Can you work these out from the drawing? Everything is in mm from the part's minimum corner. A direction names the side the tool comes from. Coordinates: 2 decimals unless noted, no trailing zeros. Loops run counter-clockwise (first coordinate to the right, second up) from the corner with the lowest first, then second, coordinate; pieces in that order, holes last. Notation, with made-up numbers: M -31.75,-37 L -9.75,-37 A11 ccw -9.75,-30 Z; hole C -7,36.5 d1. An arc over 180 degrees is marked long. Write each question's results on one line, items separated by ' | '.
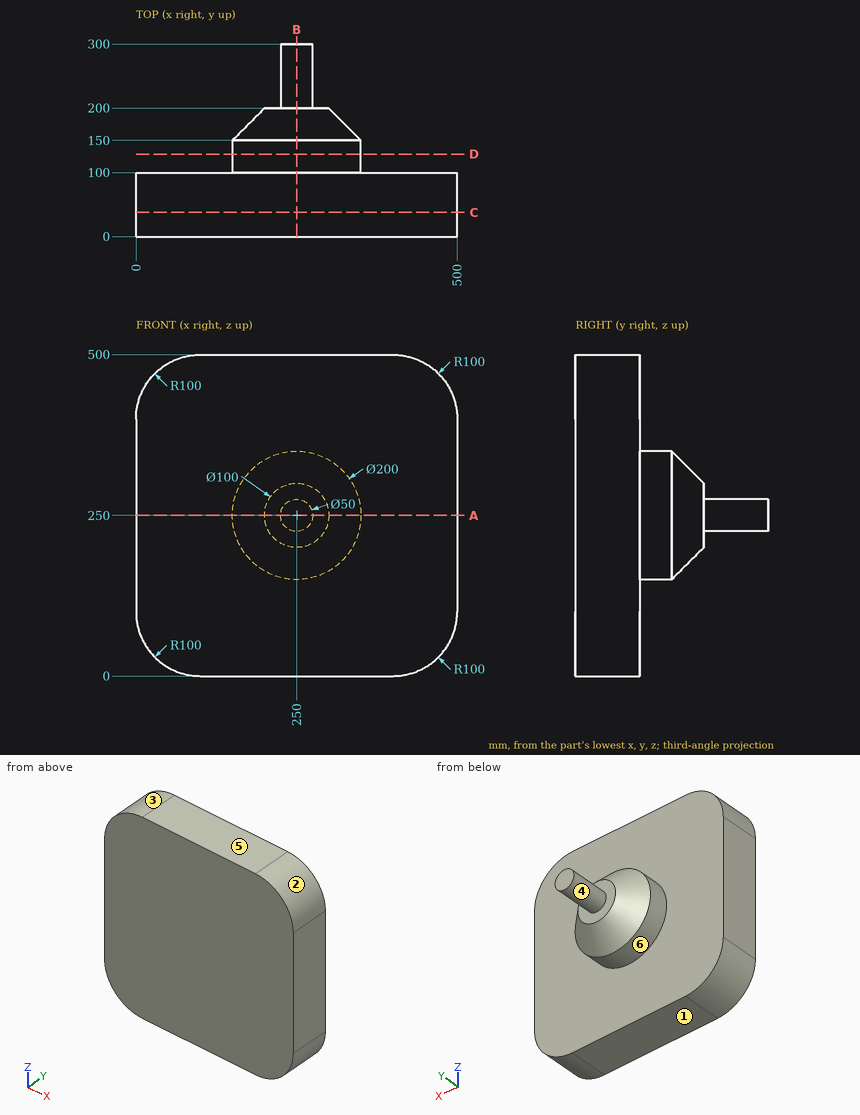
(1) If we mould it in two halves opening along X, with no side actions, what happens to the marked faces 1, 2, 3 and 4? For each: released by +X, released by -X, zero draft, split by the parting line, or undercut.
Reported:
face 1: zero draft | face 2: released by +X | face 3: released by -X | face 4: split by the parting line
(2) Imagine slicing it at B-B, the plane x = 250. List the corners of the cut face in (y, z) for me, and give its area (3 significant figures).
Reported:
outline: M 0,0 L 100,0 L 100,150 L 150,150 L 200,200 L 200,225 L 300,225 L 300,275 L 200,275 L 200,300 L 150,350 L 100,350 L 100,500 L 0,500 Z | area: 72,500 mm2
(3) Imagine slicing it at D-D, the plane y = 128.5. List the corners of the cut face in (x, z) for me.
Reported:
outline: C 250,250 d200
(4) Imagine slicing it at A-A, the plane z = 250. List the corners of the cut face in (x, y) for me.
Reported:
outline: M 0,0 L 500,0 L 500,100 L 350,100 L 350,150 L 300,200 L 275,200 L 275,300 L 225,300 L 225,200 L 200,200 L 150,150 L 150,100 L 0,100 Z
(5) Will these pins go through, and if not, where does the flat tip stop? P1, Ø12, axis at x = 190.5, z = 251, coming from the -Y side; P2, Ø1.5, axis at x = 54.5, y = 55.5, coming from the -Z side; P3, Ø4, axis at x = 233.5, z = 306.5, coming from the +Y side; P4, Ø4, axis at x = 96, z = 95, coming from the +Y side.
Reported:
P1: stops at y = 0 | P2: stops at z = 10.57 | P3: stops at y = 193.14 | P4: stops at y = 100
(6) Imagine slicing it at C-C, the plane y = 38. List the corners of the cut face in (x, z) for me.
Reported:
outline: M 0,100 A100 ccw 100,0 L 400,0 A100 ccw 500,100 L 500,400 A100 ccw 400,500 L 100,500 A100 ccw 0,400 Z
(7) Please list where these lines run through material, in increasing order: probe 1 along Z at (x, y) = (401, 18) (3 decimals); probe 2 along Y at (x, z) = (39, 78); probe 3 along Y at (x, z) = (167, 203.5). Write a range as from..to.
Reported:
probe 1: z = 0.005..499.995 | probe 2: y = 0..100 | probe 3: y = 0..154.86
(8) Which directions (+Z, -Z, +X, -X, +Y, -Y) give clear straight access to the entire face, cutting with the end or side of a thin tool? Please do the marked faces 5 and 6.
Reported:
face 5: +Z, +X, -X, +Y, -Y | face 6: +Y
